The model under review builds one solid part; all positions refer to its coordinate system, in mm. Face numbers are marked on the shaded views. A direction names the side the tool comes from. Round coordinates to 2 decimals unless told otherwise and drop trailing zeros. Order: outer loops, then holes, each group sorted by start corner. A loop starts at its lowest first (then second) coordinate and runs counter-clockwise, first axis right, second up. Notation, with made-up numbers: (52.25, -9.75) -> (82.25, -9.75) arc R28 cw to (82.25, 17.25) -> close; hole circle Ø2 at (68, -35.5). An arc over 180 degrees is marked (long way). Return JSON: item names as keys, results as strings. Group by question number.
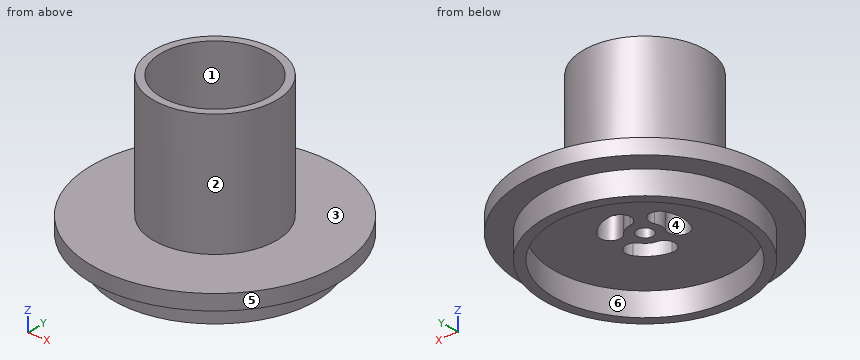
from build123d import *

# Parameters (mm, degrees)
F2_R     = 5.25
F3_DEPTH = 15.801
F4_R     = 5.25
F4_R_2   = 0.785
F5_DEPTH = 2.13


with BuildPart() as f1:
    # F0 (on Right) → F1 (revolve)
    with BuildSketch(Plane.YZ):
        Polygon((0, 13.5), (0, 0), (8.9, 0), (8.9, -2.3), (9.85, -2.3), (9.85, 0), (12, 0), (12, 1.5), (6, 1.5), (6, 13.5), align=None)
    revolve(axis=Axis((0, 0, 6.75), (0, 0, -1)))

    # F2 (on face) → F3 (cut, through all)
    with BuildSketch(Plane.XY.offset(13.5)):
        Circle(F2_R)
    extrude(amount=-F3_DEPTH, mode=Mode.SUBTRACT)

    # F4 (on face) → F5 (join)
    with BuildSketch(Plane(origin=(0, 0, 0), x_dir=(1, 0, 0), z_dir=(0, 0, -1))):
        Circle(F4_R)
        with BuildLine():
            ThreePointArc((0.3498486339, -3.5930079228), (-0.7478164186, -2.6901339379), (0.1550575663, -1.5924688855))
            ThreePointArc((0.1550575663, -1.5924688855), (0.8, -1.3856406461), (1.3015897264, -0.9305182342))
            ThreePointArc((1.3015897264, -0.9305182342), (2.7036325391, -0.6974389531), (2.9367118202, -2.0994817658))
            ThreePointArc((2.9367118202, -2.0994817658), (1.805, -3.1263517077), (0.3498486339, -3.5930079228))
        make_face(mode=Mode.SUBTRACT)
        with BuildLine():
            ThreePointArc((-3.2865604541, -1.493526157), (-3.61, 0), (-3.2865604541, 1.493526157))
            ThreePointArc((-3.2865604541, 1.493526157), (-1.9558161205, 1.9926949848), (-1.4566472927, 0.6619506513))
            ThreePointArc((-1.4566472927, 0.6619506513), (-1.6, 0), (-1.4566472927, -0.6619506513))
            ThreePointArc((-1.4566472927, -0.6619506513), (-1.9558161205, -1.9926949848), (-3.2865604541, -1.493526157))
        make_face(mode=Mode.SUBTRACT)
        Circle(F4_R_2, mode=Mode.SUBTRACT)
        with BuildLine():
            ThreePointArc((0.3498486339, 3.5930079228), (1.805, 3.1263517077), (2.9367118202, 2.0994817658))
            ThreePointArc((2.9367118202, 2.0994817658), (2.7036325391, 0.6974389531), (1.3015897264, 0.9305182342))
            ThreePointArc((1.3015897264, 0.9305182342), (0.8, 1.3856406461), (0.1550575663, 1.5924688855))
            ThreePointArc((0.1550575663, 1.5924688855), (-0.7478164186, 2.6901339379), (0.3498486339, 3.5930079228))
        make_face(mode=Mode.SUBTRACT)
    extrude(amount=-F5_DEPTH)


solid = f1.part
Item 1: Consider section A-A on y = 0. State the section outline as (x, z) points (3 decimals), plus the area to 3 significant figures.
Item 2: Insertion check: pin 1 Ø2 at (x, z) = (-3, 5) entering from -Y; pin 2 Ø8 at (x, z) = (-1, 8) entering from +Y; pin 3 Ø1.3 at (x, y) = (0, 0) entering from -Z; pin 4 Ø8 at (x, z) = (9, 3) entering from +Y. Each pin has a flat end and moves straight along its axis. Give the tip position at first contact, or say it passes through.
Item 3: Wall thickness on line 1 along X through (y, z) = (0, 1) (3 decimals); line 2 along X through (y, z) = (0, 1.55) (3 decimals); line 3 along X through (y, z) = (0, 8.75): over which ranges is each line inside the solid? List them lowest first.
Item 4: For the marked faces 5 and 6, list the 3-axis set-ups (+Z, -Z, +X, -X, +Y, -Y) from which the entire face can be reached by the end or side of a thin tool; tool diameter is ignored.
Item 5: Consider section C-C on x = 8. State the section outline as (y, z) points.
Item 6: The part is to be moulded in two halves that separate along X. For the marked faces 1, 2, 3 and 4, say which applies: +X half, -X half, draft (parallel to the pull), parting line (faces both ways), or undercut.
Item 7: Consider section B-B on z = 10.5. State the section outline as (x, y) points, plus the area to 3 significant figures.
Values:
{
 "1": {"outline": "(-12, 0) -> (-9.85, 0) -> (-9.85, -2.3) -> (-8.9, -2.3) -> (-8.9, 0) -> (-3.61, 0) -> (-3.61, 2.13) -> (-5.25, 2.13) -> (-5.25, 13.5) -> (-6, 13.5) -> (-6, 1.5) -> (-12, 1.5) -> close; (-1.6, 0) -> (-0.785, 0) -> (-0.785, 2.13) -> (-1.6, 2.13) -> close; (0.785, 0) -> (8.9, 0) -> (8.9, -2.3) -> (9.85, -2.3) -> (9.85, 0) -> (12, 0) -> (12, 1.5) -> (6, 1.5) -> (6, 13.5) -> (5.25, 13.5) -> (5.25, 2.13) -> (0.785, 2.13) -> close", "area": "57.4 mm^2"},
 "2": {"pin 1": "y = -5.66", "pin 2": "y = 6", "pin 3": "through", "pin 4": "y = 10.77"},
 "3": {"line 1": "-12 to -3.61, -1.6 to -0.785, 0.785 to 12", "line 2": "-6 to -3.61, -1.6 to -0.785, 0.785 to 6", "line 3": "-6 to -5.25, 5.25 to 6"},
 "4": {"face 5": "+Z, -Z", "face 6": "-Z"},
 "5": {"outline": "(-8.94, 0) -> (-5.75, 0) -> (-5.75, -2.3) -> (-3.9, -2.3) -> (-3.9, 0) -> (3.9, 0) -> (3.9, -2.3) -> (5.75, -2.3) -> (5.75, 0) -> (8.94, 0) -> (8.94, 1.5) -> (-8.94, 1.5) -> close"},
 "6": {"face 1": "undercut", "face 2": "parting line", "face 3": "draft", "face 4": "undercut"},
 "7": {"outline": "circle Ø12 at (0, 0); hole circle Ø10.5 at (0, 0)", "area": "26.5 mm^2"}
}
